Geometry check sheet. Reference: the model listing, model coordinates, mm. Give positions to 0.01 mm unless a question says otherwise; leave off trailing zeros. Order: outer loops, then holes, each group sorted by start corner. A loop starts at its lowest first (then second) coordinate and runs counter-clockwise, first axis right, second up. Notation, with made-up numbers: (79.25, -19) - (135.25, -19) arc R8 cw to (135.25, -10) - close; hole circle Ø1 at (60.25, 54). An arc over 180 degrees is marked (long way). Put each result on its own line as item: value. Start each with the question number.
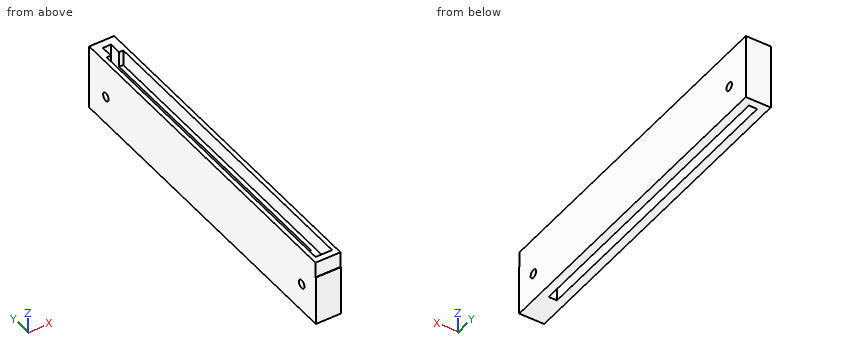
```python
from build123d import *

# Parameters (mm, degrees)
SKETCH1_W               = 3.5
SKETCH1_H               = 11.179611651
BOSS_EXTRUDE1_DEPTH     = 6.89
CUT_EXTRUDE1_DEPTH      = 10.908590231
CUT_EXTRUDE1_DEPTH_BACK = 10.908590231
SKETCH3_R               = 0.5
SKETCH4_W               = 0.5
SKETCH4_H               = 6.89
CUT_EXTRUDE2_DEPTH      = 15
SKETCH5_W               = 3
SKETCH5_H               = 6.89
BOSS_EXTRUDE2_DEPTH     = 13
SKETCH6_W               = 3
SKETCH6_H               = 6.89
BOSS_EXTRUDE3_DEPTH     = 17
SKETCH7_W               = 1.997637341
SKETCH7_H               = 38.005773156
CUT_EXTRUDE3_DEPTH      = 36.891646659
BOSS_EXTRUDE4_REACH     = 37.776
SKETCH8_W               = 6
SKETCH8_H               = 41.231307055
CUT_EXTRUDE4_DEPTH      = 36.826841099
CUT_EXTRUDE4_DEPTH_BACK = 36.826841099
SKETCH9_R               = 0.5
SKETCH10_W              = 1
SKETCH10_H              = 36.442912435
CUT_EXTRUDE5_DEPTH      = 42
CUT_EXTRUDE6_DEPTH      = 36.826841099
CUT_EXTRUDE6_DEPTH_BACK = 36.826841099
SKETCH11_R              = 0.5


with BuildPart() as part:
    # Sketch1 → Boss-Extrude1 (new body)
    with BuildSketch(Plane.XY):
        with Locations((-2.905339806, 0.611650485)):
            Rectangle(SKETCH1_W, SKETCH1_H)
    extrude(amount=BOSS_EXTRUDE1_DEPTH)

    # Sketch3 → Cut-Extrude1 (cut, two sides: drawn at the far end of the back side and taken through both)
    with BuildSketch(Plane(origin=(-1.155339806, 0, 0), x_dir=(0, 0, -1), z_dir=(1, 0, 0)).offset(-CUT_EXTRUDE1_DEPTH_BACK)):
        with Locations((-2, 4.896048014)):
            Circle(SKETCH3_R)
    extrude(amount=CUT_EXTRUDE1_DEPTH + CUT_EXTRUDE1_DEPTH_BACK, mode=Mode.SUBTRACT)

    # Sketch4 → Cut-Extrude2 (cut)
    with BuildSketch(Plane.XZ.offset(4.97815534)):
        with Locations((-4.405339806, 3.445)):
            Rectangle(SKETCH4_W, SKETCH4_H)
    extrude(amount=-CUT_EXTRUDE2_DEPTH, mode=Mode.SUBTRACT)

    # Sketch5 → Boss-Extrude2 (add)
    with BuildSketch(Plane.XZ.offset(4.97815534)):
        with Locations((-2.655339806, 3.445)):
            Rectangle(SKETCH5_W, SKETCH5_H)
    extrude(amount=BOSS_EXTRUDE2_DEPTH)

    # Sketch6 → Boss-Extrude3 (add)
    with BuildSketch(Plane.XZ.offset(17.97815534)):
        with Locations((-2.655339806, 3.445)):
            Rectangle(SKETCH6_W, SKETCH6_H)
    extrude(amount=BOSS_EXTRUDE3_DEPTH)

    # Sketch7 → Cut-Extrude3 (cut, through all)
    with BuildSketch(Plane(origin=(0, 0, 0), x_dir=(-1, 0, 0), z_dir=(0, 0, -1))):
        with Locations((2.655339806, -15.222333021)):
            Rectangle(SKETCH7_W, SKETCH7_H)
    extrude(amount=-CUT_EXTRUDE3_DEPTH, mode=Mode.SUBTRACT)

    # Boss-Extrude4: up to this face of the body (flat: up to its plane)
    boss_extrude4_end = Plane(part.part.faces().sort_by_distance((-1.155339806, -14.44187965, 3.449011069))[0])
    # Sketch8 → Boss-Extrude4 (add, up to the picked face)
    with BuildSketch(Plane.ZY.offset(4.155339806), mode=Mode.PRIVATE) as boss_extrude4_sk1:
        with Locations((2, -14.414197216)):
            Rectangle(SKETCH8_W, SKETCH8_H)
    boss_extrude4_tool1 = split(extrude(boss_extrude4_sk1.sketch, amount=-BOSS_EXTRUDE4_REACH, mode=Mode.PRIVATE), bisect_by=boss_extrude4_end, keep=Keep.BOTH, mode=Mode.PRIVATE)
    add(boss_extrude4_tool1.solids().sort_by(Axis((-4.15534, -14.414197, 2), (1, 0, 0)))[0])

    # Sketch9 → Cut-Extrude4 (cut, two sides: drawn at the far end of the back side and taken through both)
    with BuildSketch(Plane.ZY.offset(4.155339806).offset(-CUT_EXTRUDE4_DEPTH_BACK)):
        with Locations((2.4, -32.452738379)):
            Circle(SKETCH9_R)
    extrude(amount=CUT_EXTRUDE4_DEPTH + CUT_EXTRUDE4_DEPTH_BACK, mode=Mode.SUBTRACT)

    # Sketch10 → Cut-Extrude5 (cut)
    with BuildSketch(Plane(origin=(0, 0, -1), x_dir=(-1, 0, 0), z_dir=(0, 0, -1))):
        with Locations((2.655339806, -12.970585166)):
            Rectangle(SKETCH10_W, SKETCH10_H)
    extrude(amount=-CUT_EXTRUDE5_DEPTH, mode=Mode.SUBTRACT)

    # Sketch11 → Cut-Extrude6 (cut, two sides: drawn at the far end of the back side and taken through both)
    with BuildSketch(Plane.ZY.offset(4.155339806).offset(-CUT_EXTRUDE6_DEPTH_BACK)):
        with Locations((2.4, 3.176876258)):
            Circle(SKETCH11_R)
    extrude(amount=CUT_EXTRUDE6_DEPTH + CUT_EXTRUDE6_DEPTH_BACK, mode=Mode.SUBTRACT)


solid = part.part
```
Item 1: Cross-section at C-C (z = 4.5). Enter the section's corners in (x, y).
Item 2: Cross-section at A-A (z = 2.4). Enter the section's corners in (x, y), and give its area (3 significant figures).
Item 3: Thickness scan on line 1 along Y through (x, z) = (-1.5, 2.4); line 2 along X through (y, z) = (-30, 0.5); line 3 along X through (y, z) = (0, 6.5). Record the ranges inside material, lowest first.
Item 4: Gauge pin test, flat end, axial feed: pin 1 Ø0.9 at (x, z) = (-2, 6.5) entering from -Y. Record the tip position at first contact, or that the pin passes through.
Item 5: Cross-section at B-B (y = -3). Enter the section's corners in (x, z), and give its area (3 significant figures).
Recorded:
1. outline: (-4.16, -35.03) - (-1.16, -35.03) - (-1.16, 6.2) - (-4.16, 6.2) - close; hole (-3.16, -31.19) - (-2.16, -31.19) - (-2.16, 5.25) - (-3.16, 5.25) - close
2. outline: (-4.16, -35.03) - (-1.16, -35.03) - (-1.16, -32.95) - (-4.16, -32.95) - close; (-4.16, -31.95) - (-1.16, -31.95) - (-1.16, 2.68) - (-2.16, 2.68) - (-2.16, -31.19) - (-3.16, -31.19) - (-3.16, 2.68) - (-4.16, 2.68) - close; (-4.16, 3.68) - (-3.16, 3.68) - (-3.16, 5.25) - (-2.16, 5.25) - (-2.16, 3.68) - (-1.16, 3.68) - (-1.16, 6.2) - (-4.16, 6.2) - close
2. area: 82.3 mm^2
3. line 1: y = -35.03 to -32.95, -31.95 to 2.68, 3.68 to 6.2
3. line 2: x = -4.16 to -3.16, -2.16 to -1.16
3. line 3: x = -4.16 to -3.65, -1.66 to -1.16
4. pin 1: stops at y = -34.98
5. outline: (-4.16, -1) - (-3.16, -1) - (-3.16, 5) - (-3.65, 5) - (-3.65, 6.89) - (-4.16, 6.89) - close; (-2.16, -1) - (-1.16, -1) - (-1.16, 6.89) - (-1.66, 6.89) - (-1.66, 5) - (-2.16, 5) - close
5. area: 13.9 mm^2
